```python
from build123d import *

# Parameters (mm, degrees)
SKETCH1_W           = 5
SKETCH1_H           = 6.5
EXTRUDE1_DEPTH      = 1.175
EXTRUDE1_DEPTH_BACK = 1.175
CUT_EXTRUDE1_START  = -1
SKETCH2_OUTSIDE_W   = 8.706
SKETCH2_OUTSIDE_H   = 6.056
SKETCH2_OUTSIDE_W_2 = 4.7
SKETCH2_OUTSIDE_H_2 = 2.05
CUT_EXTRUDE1_DEPTH  = 1
SKETCH3_W           = 4
SKETCH3_H           = 1.35
CUT_EXTRUDE2_DEPTH  = 4


with BuildPart() as part:
    # Sketch1 → Extrude1 (new body, two sides)
    with BuildSketch(Plane.XY) as extrude1_sk:
        Rectangle(SKETCH1_W, SKETCH1_H)
    extrude(amount=EXTRUDE1_DEPTH)
    extrude(extrude1_sk.sketch, amount=-EXTRUDE1_DEPTH_BACK)

    # Sketch2 outside → Cut-Extrude1 (cut)
    with BuildSketch(Plane(origin=(0, 3.25, 0), x_dir=(1, 0, 0), z_dir=(0, 1, 0)).offset(CUT_EXTRUDE1_START)):
        Rectangle(SKETCH2_OUTSIDE_W, SKETCH2_OUTSIDE_H)
        Rectangle(SKETCH2_OUTSIDE_W_2, SKETCH2_OUTSIDE_H_2, mode=Mode.SUBTRACT)
    extrude(amount=-CUT_EXTRUDE1_DEPTH, mode=Mode.SUBTRACT)

    # Sketch3 → Cut-Extrude2 (cut)
    with BuildSketch(Plane.XZ.offset(3.25)):
        Rectangle(SKETCH3_W, SKETCH3_H)
    extrude(amount=-CUT_EXTRUDE2_DEPTH, mode=Mode.SUBTRACT)


solid = part.part
```
Part model, mm, in its own coordinate system. A direction names the side the tool comes from. Give positions to 0.01 mm unless a question says otherwise; leave off trailing zeros. Write each loop counter-clockwise with the first axis right and the second up, starting at its lowest first coordinate (ties: lowest second). Pieces come first, ordered by that corner, then holes. Notation, with made-up numbers: (4, 50) -> (54, 50) arc R26 cw to (54, 80) -> close; hole circle Ø9 at (53, 29.5). An arc over 180 degrees is marked (long way). Put each result on its own line as item: value. Start each with the question number.
Item 1: Wall check: L1, parallel to X at y = -2.5, z = 0.35; L2, parallel to Z at x = 1.55, y = -1 (3 decimals); L3, parallel to Y at x = 1, z = 0.05. Give the ranges that are in metal, low to high. Write a range as [from, to].
Item 2: Pull direction Y, two halves, no side cores. Call faces 1 (the face through (2.5, 3, 0)), 2 (the face through (-2.35, 2, 0)), 3 (the face through (0, 0.75, 0)): pulls with the +Y half, pulls with the -Y half, needs draft (parallel to the pull), parting line crosses it, or undercut.
Item 3: Cut at B-B (y = 0.25). List the corners of the cut face in (x, z) (3 decimals), then the cut area to 3 significant figures.
Item 4: Cut at D-D (x = 2.15). List the corners of the cut face in (y, z) (3 decimals).
Item 5: Cut at A-A (z = -0.5). List the corners of the cut face in (x, y).
Item 6: Cut at C-C (x = -1.2). List the corners of the cut face in (y, z) (3 decimals), then the cut area to 4 significant figures.
Item 7: Which spindle directions (+Z, -Z, +X, -X, +Y, -Y) get a long thin tool onto all of the face, cutting with end or side? Do faces 4 (the face through (0, -1, 1.175)), 5 (the face through (2.35, 2, 0)), 6 (the face through (-2.5, -1, 0)), 7 (the face through (-2, -1, 0)), 8 (the face through (0, 2, -1.025)). Say none if no direction does.
Item 8: Pin check, flat tip, straight feed: pin 1 Ø1.2 at (x, z) = (1, 0) entering from -Y. Stop position of the tip, or through.
Answer list:
1. L1: x = [-2.5, -2], [2, 2.5]
1. L2: z = [-1.175, -0.675], [0.675, 1.175]
1. L3: y = [0.75, 3.25]
2. face 1: needs draft
2. face 2: undercut
2. face 3: pulls with the -Y half
3. outline: (-2.5, -1.175) -> (2.5, -1.175) -> (2.5, 1.175) -> (-2.5, 1.175) -> close; hole (-2, -0.675) -> (2, -0.675) -> (2, 0.675) -> (-2, 0.675) -> close
3. area: 6.35 mm2
4. outline: (-3.25, -1.175) -> (1.25, -1.175) -> (1.25, -1.025) -> (2.25, -1.025) -> (2.25, -1.175) -> (3.25, -1.175) -> (3.25, 1.175) -> (2.25, 1.175) -> (2.25, 1.025) -> (1.25, 1.025) -> (1.25, 1.175) -> (-3.25, 1.175) -> close
5. outline: (-2.5, -3.25) -> (-2, -3.25) -> (-2, 0.75) -> (2, 0.75) -> (2, -3.25) -> (2.5, -3.25) -> (2.5, 1.25) -> (2.35, 1.25) -> (2.35, 2.25) -> (2.5, 2.25) -> (2.5, 3.25) -> (-2.5, 3.25) -> (-2.5, 2.25) -> (-2.35, 2.25) -> (-2.35, 1.25) -> (-2.5, 1.25) -> close
6. outline: (-3.25, -1.175) -> (1.25, -1.175) -> (1.25, -1.025) -> (2.25, -1.025) -> (2.25, -1.175) -> (3.25, -1.175) -> (3.25, 1.175) -> (2.25, 1.175) -> (2.25, 1.025) -> (1.25, 1.025) -> (1.25, 1.175) -> (-3.25, 1.175) -> (-3.25, 0.675) -> (0.75, 0.675) -> (0.75, -0.675) -> (-3.25, -0.675) -> close
6. area: 9.575 mm2
7. face 4: +Z, +X, -X, +Y, -Y
7. face 5: +Z, -Z, +X
7. face 6: +Z, -Z, -X, +Y, -Y
7. face 7: -Y
7. face 8: -Z, +X, -X
8. pin 1: stops at y = 0.75
